For this review, take the finished solid that the model builds, in its own axes (mm). A direction names the side the tool comes from. Coordinates: 2 decimals unless noted, no trailing zeros. Order: outer loops, then holes, each group sorted by start corner. A loop starts at its lowest first (then second) coordinate and runs counter-clockwise, first axis right, second up. Notation, with made-up numbers: M 40.5,66 L 75.5,66 A24 ccw 75.5,85 Z; hole C 8.25,8.5 d7. An arc over 180 degrees is marked long. Use one line per item in the form item = value. Start each with the question number.
Autodesk Inventor part; units mm, degrees
ref_plane "YZ Plane" through (0, 0, 0) normal (1, 0, 0) x (0, 1, 0)
ref_plane "XZ Plane" through (0, 0, 0) normal (0, 1, 0) x (-1, 0, 0)
ref_plane "XY Plane" through (0, 0, 0) normal (0, 0, 1) x (1, 0, 0)
sketch "スケッチ1" plane through (0, 0, 0) normal (0, 0, 1) x (1, 0, 0)
  line L0 (0, 0) -> (-81, 0)
  line L1 (-81, 0) -> (-81, 17)
  line L2 (-81, 17) -> (0, 17)
  line L3 (0, 17) -> (0, 0)
  line L4 (-81, 8.5) -> (0, 8.5)
  circle A0 centre (-81, 8.5) radius 23.5
  point P0 (-59.0911, 17)
  point P1 (-59.0911, 0)
  dimension "d0" = 17
  dimension "d28" = 47
  dimension "d29" = 81
extrude "押し出し1" add sketch "スケッチ1" along normal blind 3
sketch "スケッチ2" plane through (0, 0, 3) normal (0, 0, 1) x (1, 0, 0)
  line L0 (0, 0) -> (0, 17)
  line L1 (0, 8.5) -> (-59.0911, 8.5)
  line L2 (0, 17) -> (-59.0911, 17)
  line L3 (-5, 17) -> (-5, 0)
  line L4 (-35, 17) -> (-35, 0)
  line L5 (-59.0911, 0) -> (0, 0)
  arc A0 (-59.0911, 17) -> (-59.0911, 0) centre (-81, 8.5) ccw
  line L6 (-59.0911, 17) -> (-59.0911, 0)
  point P0 (-5, 14.5)
  point P1 (-35, 14.5)
  point P2 (-5, 2.5)
  point P3 (-35, 2.5)
  dimension "d4" = 5
  dimension "d5" = 30
  dimension "d6" = 6
  dimension "d7" = 6
hole "穴1" at (-5, 14.5, 3) at (-35, 14.5, 3) at (-35, 2.5, 3) at (-5, 2.5, 3) direction (0, 0, -1) diameter 3.1 depth 20 tip angle 118
sketch "スケッチ5" plane through (0, 0, 3) normal (0, 0, 1) x (1, 0, 0)
  arc A0 (-59.0911, 17) -> (-59.0911, 0) centre (-81, 8.5) ccw
  line L0 (-59.0911, 0) -> (0, 0)
  line L1 (0, 0) -> (0, 17)
  circle A1 centre (-81, 8.5) radius 19
  line L2 (-81, 8.5) -> (-81, 27.5)
  line L3 (-81, 8.5) -> (-94.435, 21.935)
  point P0 (-94.435, -4.935)
  point P1 (-67.565, -4.935)
  point P2 (-67.565, 21.935)
  dimension "d80" = 38
  dimension "d81" = 45
  dimension "d84" = 360
hole "穴3" at (-67.565, 21.935, 3) at (-67.565, -4.935, 3) at (-94.435, -4.935, 3) at (-94.435, 21.935, 3) direction (0, 0, -1) diameter 3.1 end through all
sketch "スケッチ6" plane through (0, 0, 3) normal (0, 0, 1) x (1, 0, 0)
  arc A0 (-59.0911, 17) -> (-59.0911, 0) centre (-81, 8.5) ccw
  circle A1 centre (-81, 8.5) radius 6
  point P0 (0, 0)
  dimension "d43" = 12
extrude "押し出し3" cut sketch "スケッチ6" against normal blind 3
sketch "スケッチ7" plane through (0, 0, 3) normal (0, 0, 1) x (1, 0, 0)
  circle A0 centre (-94.435, -4.935) radius 1.55
  circle A1 centre (-67.565, -4.935) radius 1.55
  circle A2 centre (-67.565, -4.935) radius 3
  circle A3 centre (-94.435, -4.935) radius 3
  circle A4 centre (-94.435, 21.935) radius 1.55
  circle A5 centre (-94.435, 21.935) radius 3
  circle A6 centre (-67.565, 21.935) radius 1.55
  circle A7 centre (-67.565, 21.935) radius 3
  point P0 (0, 0)
  dimension "d86" = 6
  dimension "d87" = 6
  dimension "d88" = 6
  dimension "d89" = 6
extrude "押し出し4" cut sketch "スケッチ7" against normal blind 2 contours A0 | A1 | A2 | A3 | A4 | A5 | A6 | A7
sketch "スケッチ8" plane through (0, 0, 3) normal (0, 0, 1) x (1, 0, 0)
  line L0 (-81, 8.5) -> (-81, 30.5)
  line L1 (-81, 8.5) -> (-20.8346, 112.7096)
  line L2 (-77, 15.4282) -> (-20.8346, 112.7096)
  circle A0 centre (-81, 8.5) radius 22
  circle A1 centre (-81, 8.5) radius 8
  line L3 (0, 17) -> (-59.0911, 17)
  line L4 (-57, 17) -> (-57, -1.5)
  line L5 (-38, 17) -> (-38, 0)
  line L6 (-59.0911, 0) -> (0, 0)
  line L7 (-32, 17) -> (-32, 0)
  circle A2 centre (-35, 14.5) radius 1.55
  line L8 (-10, 17) -> (-10, 0)
  line L9 (0, 0) -> (0, 17)
  line L10 (-57, 3) -> (0, 3)
  line L11 (-57, 14) -> (0, 14)
  line L12 (-57, 3) -> (-38, 14)
  line L13 (-57, 4.7332) -> (-40.9938, 14)
  line L14 (-54.0062, 3) -> (-38, 12.2668)
  line L15 (-32, 14) -> (-10, 3)
  line L16 (-32, 12.3229) -> (-13.3541, 3)
  line L17 (-28.6459, 14) -> (-10, 4.6771)
  line L18 (-85, 15.4282) -> (-141.1654, 112.7096)
  line L19 (-87.9282, 4.5) -> (-185.2096, -51.6654)
  line L20 (-81, 8.5) -> (-185.2096, 68.6654)
  line L21 (-77, 1.5718) -> (-20.8346, -95.7096)
  line L22 (-81, 8.5) -> (-141.1654, -95.7096)
  line L23 (-74.0718, 12.5) -> (23.2096, 68.6654)
  line L24 (-81, 8.5) -> (23.2096, -51.6654)
  circle A3 centre (-81, 8.5) radius 6
  point P0 (-10, 14)
  point P1 (-32, 3)
  point P2 (-38, 3)
  point P3 (-87.9282, 12.5)
  point P4 (-85, 1.5718)
  point P5 (-74.0718, 4.5)
  point P6 (-85, 1.5718)
  point P7 (-92, -10.5526)
  point P8 (-70, -10.5526)
  point P9 (-77, 1.5718)
  point P10 (-74.0718, 4.5)
  point P11 (-61.9474, -2.5)
  point P12 (-61.9474, 19.5)
  point P13 (-74.0718, 12.5)
  point P14 (-92, 27.5526)
  point P15 (-85, 15.4282)
  point P16 (-70, 27.5526)
  point P17 (-87.9282, 12.5)
  point P18 (-100.0526, 19.5)
  point P19 (-100.0526, -2.5)
  point P20 (-87.9282, 4.5)
  dimension "d57" = 44
  dimension "d69" = 16
  dimension "d52" = 30
  dimension "d58" = 24
  dimension "d59" = 3
  dimension "d60" = 3
  dimension "d61" = 10
  dimension "d62" = 3
  dimension "d63" = 3
  dimension "d64" = 1.5
  dimension "d66" = 1.5
  dimension "d67" = 1.5
  dimension "d68" = 1.5
  dimension "d74" = 360
extrude "押し出し5" cut sketch "スケッチ8" against normal blind 3 contours A1 L18 A0 L0 | L0 A0 L1 A1 | A1 L19 A0 L20 | A1 L21 A0 L22 | A1 L23 A0 L24 | L8 L17 L11 | L16 L10 L7 | L11 L13 L4 | L5 L10 L14
fillet "フィレット1" radius 1.5 16 edges at (-100.0526, 19.5, 1.5) (-87.9282, 12.5, 1.5) (-85, 15.4282, 1.5) (-92, 27.5526, 1.5) (-70, 27.5526, 1.5) (-77, 15.4282, 1.5) (-74.0718, 12.5, 1.5) (-61.9474, 19.5, 1.5) (-74.0718, 4.5, 1.5) (-61.9474, -2.5, 1.5) (-70, -10.5526, 1.5) (-77, 1.5718, 1.5) (-85, 1.5718, 1.5) (-92, -10.5526, 1.5) (-87.9282, 4.5, 1.5) (-100.0526, -2.5, 1.5)
fillet "フィレット2" radius 13 2 edges at (-59.0911, 17, 1.5) (-59.0911, 0, 1.5)
fillet "フィレット3" radius 5 2 edges at (0, 17, 1.5) (0, 0, 1.5)
sketch "スケッチ9" plane through (0, 0, 3) normal (0, 0, 1) x (1, 0, 0)
  line L0 (-51.5042, 0) -> (-5, 0)
  line L1 (-27.5, 0) -> (-27.5, 17)
  line L2 (-5, 17) -> (-51.5042, 17)
  line L3 (-47.5, 0) -> (-47.5, 17)
  line L4 (0, 5) -> (0, 12)
  point P0 (0, 0)
  point P1 (-47.5, 17)
  point P2 (-47.5, 0)
  dimension "d90" = 27.5
  dimension "d91" = 20
extrude "押し出し6" cut sketch "スケッチ9" against normal blind 1.5
properties part number "link2plate4" material "アルミニウム 6061"
1. Consider section C-C, the plane z = 2.15. Give the number of separate pieces and of enclosed holes in the cut face, plus the area to 3 significant figures.
2. To check wall thickness, follow line 1 (Y direction, x = -53.5, z = 0.3); line 2 (X direction, y = 24, z = 2); line 3 (X direction, y = -4, z = 1.8). State the ranges of each line that lie inside material, in increasing order.
3. Consider section B-B, the plane x = -35. Write out the cut boundary in (y, z).
4. The part is to be moulded in two halves that separate along X. For faces 4 (the cylindrical face through (-89, 8.5, 1.5)), 5 (the flat face through (-74, 10, 3)), 6 (the cylindrical face through (-2, 1, 2)), say which applies: pulls with the +X half, pulls with the -X half, needs draft (parallel to the pull), parting line crosses it, or undercut.
5. Consider section A-A, the plane x = -81. Write out the cut boundary in (y, z), plus the area to 3 significant figures.
6. Tool access review of faces 1 (the cylindrical face through (-1, 15, 2)), 2 (the flat face through (-66, 21, 1)), 3 (the cylindrical face through (-77.093, 15.965, 1.479)): name each direction out of +Z, -Z, +X, -X, +Y, -Y from which nothing blocks a thin tool from reaching the whole face with its end or side.
7. For pin 1 Ø1.2 at (y, z) = (16, 2.5) entering from -X; pin 2 Ø0.9 at (y, z) = (10, 2) entering from -X; pin 3 Ø1.9 at (x, y) = (-35, 14.5) entering from +Z; pin 4 Ø1.2 at (y, z) = (1.5, 2.5) entering from -X, all flat-tipped, find the tip position at first contact; note any pin that passes through.
Answers follow:
q1.separate_pieces = 2
q1.enclosed_holes = 11
q1.area = 1,060 mm²
q2.line_1 = -0.15 to 3, 3.29 to 6.76, 14 to 17.15
q2.line_2 = -98.66 to -96.61, -92.26 to -89.95, -72.05 to -69.74, -65.39 to -63.34
q2.line_3 = -100.9 to -97.29, -91.58 to -88.22, -73.78 to -70.42, -64.71 to -60.89
q3.outline = M 0,0 L 0.95,0 L 0.95,1.5 L 0,1.5 Z; M 4.05,0 L 12.95,0 L 12.95,1.5 L 4.05,1.5 Z; M 16.05,0 L 17,0 L 17,1.5 L 16.05,1.5 Z
q4.face_4 = undercut
q4.face_5 = needs draft
q4.face_6 = pulls with the +X half
q5.outline = M -15,0 L -13.5,0 L -13.5,3 L -15,3 Z; M 0.5,0 L 2.5,0 L 2.5,3 L 0.5,3 Z; M 14.5,0 L 16.5,0 L 16.5,3 L 14.5,3 Z; M 30.5,0 L 32,0 L 32,3 L 30.5,3 Z
q5.area = 21.0 mm²
q6.face_1 = +Z, -Z, +X, +Y
q6.face_2 = +Z
q6.face_3 = +Z, -Z
q7.pin_1 = -103.46
q7.pin_2 = -104.48
q7.pin_3 = through
q7.pin_4 = -103.61
